```python
from build123d import *

# Parameters (mm, degrees)
F0_R     = 5.08
F1_DEPTH = 0.762
F2_R     = 5.08
F3_DEPTH = 4.191
F4_W     = 60.96
F4_H     = 27.686
F5_DEPTH = 1.8796
F7_DEPTH = 13.9319
F8_DEPTH = 9.525


with BuildPart() as f1:
    # F0 (on Top) → F1 (new body)
    with BuildSketch(Plane.XY):
        with BuildLine():
            Line((33.401, 19.685), (-33.401, 19.685))
            ThreePointArc((-33.401, 19.685), (-35.646064, 18.755064), (-36.576, 16.51))
            Line((-36.576, 16.51), (-36.576, -16.51))
            ThreePointArc((-36.576, -16.51), (-35.646064, -18.755064), (-33.401, -19.685))
            Line((-33.401, -19.685), (33.401, -19.685))
            ThreePointArc((33.401, -19.685), (35.646064, -18.755064), (36.576, -16.51))
            Line((36.576, -16.51), (36.576, 16.51))
            ThreePointArc((36.576, 16.51), (35.646064, 18.755064), (33.401, 19.685))
        make_face()
        Circle(F0_R, mode=Mode.SUBTRACT)
    extrude(amount=F1_DEPTH)

    # F2 (on Top) → F3 (join)
    with BuildSketch(Plane.XY):
        with BuildLine():
            Line((33.655, 19.05), (-33.655, 19.05))
            ThreePointArc((-33.655, 19.05), (-35.271446, 18.380446), (-35.941, 16.764))
            Line((-35.941, 16.764), (-35.941, -16.764))
            ThreePointArc((-35.941, -16.764), (-35.271446, -18.380446), (-33.655, -19.05))
            Line((-33.655, -19.05), (33.655, -19.05))
            ThreePointArc((33.655, -19.05), (35.271446, -18.380446), (35.941, -16.764))
            Line((35.941, -16.764), (35.941, 16.764))
            ThreePointArc((35.941, 16.764), (35.271446, 18.380446), (33.655, 19.05))
        make_face()
        Circle(F2_R, mode=Mode.SUBTRACT)
    extrude(amount=F3_DEPTH)

    # F4 (on Top) → F5 (cut)
    with BuildSketch(Plane.XY):
        Rectangle(F4_W, F4_H)
    extrude(amount=F5_DEPTH, mode=Mode.SUBTRACT)

    # F6 (on Front) → F7 (join, symmetric)
    with BuildSketch(Plane.XZ):
        Polygon((-33.1343, 0), (-34.4805, 0), (-34.4805, -1.3462), (-35.1155, -1.3462), (-33.6423, -6.35), (-33.1343, -6.35), align=None)
        Polygon((33.1343, 0), (33.1343, -6.35), (33.6423, -6.35), (35.1155, -1.3462), (34.4805, -1.3462), (34.4805, 0), align=None)
    extrude(amount=F7_DEPTH, both=True)

    # F6 (on Front) → F8 (cut, symmetric)
    with BuildSketch(Plane.XZ):
        Polygon((-33.1343, 0), (-34.4805, 0), (-34.4805, -1.3462), (-35.1155, -1.3462), (-33.6423, -6.35), (-33.1343, -6.35), align=None)
        Polygon((33.1343, 0), (33.1343, -6.35), (33.6423, -6.35), (35.1155, -1.3462), (34.4805, -1.3462), (34.4805, 0), align=None)
    extrude(amount=F8_DEPTH, both=True, mode=Mode.SUBTRACT)


solid = f1.part
```
The listing builds one solid part. Answer for the finished solid, in the listing's coordinates (mm). A direction names the side the tool comes from. Give positions to 0.01 mm unless a question says otherwise; leave off trailing zeros. Order: outer loops, then holes, each group sorted by start corner. A loop starts at its lowest first (then second) coordinate and runs counter-clockwise, first axis right, second up.
1) Given P1, Ø2, axis at x = -34.5, z = -2.5, coming from the +Y side; P2, Ø2, axis at x = -3, z = 2, coming from the -Y side; P3, Ø2, axis at y = 11, z = -2.5, coming from the -X side, each flat-ended and moving along its own axis, determine where each tip first touches the part or whether it passes through.
Reported:
P1: stops at y = 13.93
P2: stops at y = -19.05
P3: stops at x = -35.07
2) Determine the mould class of faces 6 (the face through (-34.39, 11.76, -3.81)), 7 (the face through (0, 13.843, 1)), 8 (the face through (-35.6, 18.8, 0.4)), 9 (the face through (30.48, 0, 1)) for opening direction Y: pulls with the +Y half, pulls with the -Y half, needs draft (parallel to the pull), parting line crosses it, or undercut.
Reported:
face 6: needs draft
face 7: undercut
face 8: pulls with the +Y half
face 9: undercut
3) For faces 1 (the face through (0, 19.05, 2)), 2 (the face through (34, -9.525, -2)), 3 (the face through (0, -13.843, 1)), 4 (the face through (-35.25, 18.4, 2.45)), 5 (the face through (-34.48, 12, -1)), determine the directions among +Z, -Z, +X, -X, +Y, -Y from which every point of the face is accessible in a straight line to the end or side of a thin tool.
Reported:
face 1: +Z, +X, -X, +Y
face 2: -Z, +X, -X
face 3: -Z
face 4: +Z, -X, +Y
face 5: -X, +Y, -Y
4) Find section C-C on z = 3. Write down the section's boundary in (x, y) (3 decimals), then the cut area to 3 significant figures.
Reported:
outline: (-35.941, -16.764) arc R2.286 ccw to (-33.655, -19.05) - (33.655, -19.05) arc R2.286 ccw to (35.941, -16.764) - (35.941, 16.764) arc R2.286 ccw to (33.655, 19.05) - (-33.655, 19.05) arc R2.286 ccw to (-35.941, 16.764) - close; hole circle Ø10.16 at (0, 0)
area: 2,650 mm2
5) Find section D-D on z = -2.5. Write down the section's boundary in (x, y) (3 decimals), then the cut area to 3 significant figures.
Reported:
outline: (-34.776, -13.932) - (-33.134, -13.932) - (-33.134, -9.525) - (-34.776, -9.525) - close; (-34.776, 9.525) - (-33.134, 9.525) - (-33.134, 13.932) - (-34.776, 13.932) - close; (33.134, -13.932) - (34.776, -13.932) - (34.776, -9.525) - (33.134, -9.525) - close; (33.134, 9.525) - (34.776, 9.525) - (34.776, 13.932) - (33.134, 13.932) - close
area: 28.9 mm2
6) Consider line 1 along X through (y, z) = (0, 2.5); line 2 along Y through (x, z) = (-12.5, 0.25) (3 decimals); line 3 along Y through (x, z) = (23, 1). Determine where each line is inside the solid, lowest interval first.
Reported:
line 1: x = -35.94 to -5.08, 5.08 to 35.94
line 2: y = -19.685 to -13.843, 13.843 to 19.685
line 3: y = -19.05 to -13.84, 13.84 to 19.05
7) Find section A-A on y = 0. Write down the section's boundary in (x, z), then the cut area to 3 significant figures.
Reported:
outline: (-36.58, 0) - (-30.48, 0) - (-30.48, 1.88) - (-5.08, 1.88) - (-5.08, 4.19) - (-35.94, 4.19) - (-35.94, 0.76) - (-36.58, 0.76) - close; (5.08, 1.88) - (30.48, 1.88) - (30.48, 0) - (36.58, 0) - (36.58, 0.76) - (35.94, 0.76) - (35.94, 4.19) - (5.08, 4.19) - close
area: 164 mm2
8) Find section B-B on x = 0. Write down the section's boundary in (y, z) (3 decimals), then the cut area to 3 significant figures.
Reported:
outline: (-19.685, 0) - (-13.843, 0) - (-13.843, 1.88) - (-5.08, 1.88) - (-5.08, 4.191) - (-19.05, 4.191) - (-19.05, 0.762) - (-19.685, 0.762) - close; (5.08, 1.88) - (13.843, 1.88) - (13.843, 0) - (19.685, 0) - (19.685, 0.762) - (19.05, 0.762) - (19.05, 4.191) - (5.08, 4.191) - close
area: 85.1 mm2
